Geometry: final body of the model. Coordinates: model frame, mm. Coordinates: 2 decimals unless noted, no trailing zeros. Write each loop counter-clockwise with the first axis right and the second up, starting at its lowest first coordinate (ties: lowest second). Pieces come first, ordered by that corner, then holes. Notation, with made-up numbers: M 18.5,64.25 L 38.5,64.25 A25 ccw 38.5,78.25 Z; hole C -0.5,17 d10. An arc over 180 degrees is marked long. Write item = value, one per line. Start each with the question number.
Item 1: Section B-B on x = 1.75. Output: boundary loops of the cut face in (y, z).
Item 2: First-contact query: pin 1 Ø4 at (y, z) = (39, 1) entering from +X. Flat tip, straight axial feed; report the tip coordinate or a pass-through.
Item 3: Section C-C on y = -40. Output: boundary loops of the cut face in (x, z), plus the area to 3 significant figures.
Item 4: Section A-A on z = 0. Output: boundary loops of the cut face in (x, y), plus the area to 3 significant figures.
Item 5: Ray query, L1, parallel to Z at x = 1.9, y = 40; L2, parallel to Y at x = 1.1, z = 2.25; L3, parallel to Y at x = 1.85, z = 0.75. Return the intervals inside material, ascending. Write a range as [from, to].
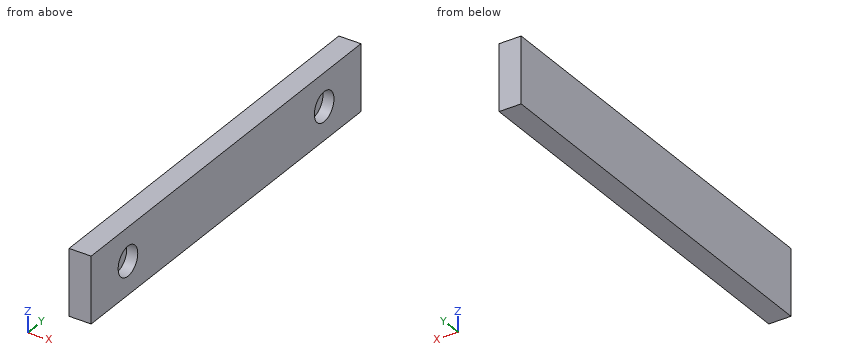
from build123d import *

# Parameters (mm, degrees)
F0_W     = 110
F0_H     = 18
F1_DEPTH = 3
F2_R     = 4
F3_DEPTH = 3


with BuildPart() as f1:
    # F0 (on Right) → F1 (new body, symmetric)
    with BuildSketch(Plane.YZ):
        Rectangle(F0_W, F0_H)
    extrude(amount=F1_DEPTH, both=True)

    # F2 (on face) → F3 (cut)
    with BuildSketch(Plane.YZ.offset(3)):
        with Locations((-40, 0)):
            Circle(F2_R)
        with Locations((40, 0)):
            Circle(F2_R)
    extrude(amount=-F3_DEPTH, mode=Mode.SUBTRACT)


solid = f1.part
Responses:
q1.outline = M -55,-9 L 55,-9 L 55,9 L -55,9 Z; hole C -40,0 d8; hole C 40,0 d8
q2.pin_1 = 0
q3.outline = M -3,-9 L 3,-9 L 3,-4 L 0,-4 L 0,4 L 3,4 L 3,9 L -3,9 Z
q3.area = 84.0 mm²
q4.outline = M -3,-55 L 3,-55 L 3,-44 L 0,-44 L 0,-36 L 3,-36 L 3,36 L 0,36 L 0,44 L 3,44 L 3,55 L -3,55 Z
q4.area = 612 mm²
q5.L1 = [-9, -4], [4, 9]
q5.L2 = [-55, -43.31], [-36.69, 36.69], [43.31, 55]
q5.L3 = [-55, -43.93], [-36.07, 36.07], [43.93, 55]
